from build123d import *

# Parameters (mm, degrees)
EXTRUDE_1_DEPTH          = 7
SKETCH_2_R               = 3.5
CUT_EXTRUDE_2_DEPTH      = 7
FILLET_1_R               = 7
EXTRUDE_2_DEPTH          = 29
SKETCH_4_R               = 7
CUT_EXTRUDE_3_DEPTH      = 30
CUT_EXTRUDE_4_DEPTH      = 6
SKETCH_6_R               = 4
CUT_EXTRUDE_5_DEPTH      = 17
CUT_EXTRUDE_5_DEPTH_BACK = 15
EXTRUDE_3_DEPTH          = 5


with BuildPart() as part:
    # 草图1 → 凸台-拉伸1 (new body)
    with BuildSketch(Plane(origin=(0, 0, 0), x_dir=(1, 0, 0), z_dir=(0, 1, 0))):
        Polygon((0, 0), (27, 0), (27, -37), (-27, -37), (-27, 0), align=None)
    extrude(amount=EXTRUDE_1_DEPTH)

    # 草图2 → 切除-拉伸2 (cut)
    with BuildSketch(Plane(origin=(0, 0, 0), x_dir=(1, 0, 0), z_dir=(0, 1, 0))):
        with Locations((-20, -30)):
            Circle(SKETCH_2_R)
        with Locations((20, -30)):
            Circle(SKETCH_2_R)
    extrude(amount=CUT_EXTRUDE_2_DEPTH, mode=Mode.SUBTRACT)

    # 圆角1
    fillet_1_edges = [part.edges().sort_by_distance(p)[0] for p in [
        (27, 3.5, 37),
        (-27, 3.5, 37),
    ]]
    fillet(fillet_1_edges, radius=FILLET_1_R)

    # 草图3 → 凸台-拉伸2 (add)
    with BuildSketch(Plane(origin=(0, 0, 0), x_dir=(1, 0, 0), z_dir=(0, 1, 0))):
        with BuildLine():
            Line((0, 0), (-12, 0))
            Line((-12, 0), (-12, -14))
            ThreePointArc((-12, -14), (0, -26), (12, -14))
            Line((12, -14), (12, 0))
            Line((12, 0), (0, 0))
        make_face()
    extrude(amount=EXTRUDE_2_DEPTH)

    # 草图4 → 切除-拉伸3 (cut, through all)
    with BuildSketch(Plane(origin=(0, 29, 0), x_dir=(1, 0, 0), z_dir=(0, 1, 0))):
        with Locations((0, -14)):
            Circle(SKETCH_4_R)
    extrude(amount=-CUT_EXTRUDE_3_DEPTH, mode=Mode.SUBTRACT)

    # 草图5 → 切除-拉伸4 (cut)
    with BuildSketch(Plane(origin=(0, 29, 0), x_dir=(1, 0, 0), z_dir=(0, 1, 0))):
        with BuildLine():
            Line((-7, -14), (-12, -14))
            ThreePointArc((-12, -14), (0, -26), (12, -14))
            Line((12, -14), (7, -14))
            ThreePointArc((7, -14), (0, -21), (-7, -14))
        make_face()
    extrude(amount=-CUT_EXTRUDE_4_DEPTH, mode=Mode.SUBTRACT)

    # 草图6 → 切除-拉伸5 (cut, two sides)
    with BuildSketch(Plane.XY.offset(14)) as cut_extrude_5_sk:
        with Locations((0, 23)):
            Circle(SKETCH_6_R)
    extrude(amount=CUT_EXTRUDE_5_DEPTH, mode=Mode.SUBTRACT)
    extrude(cut_extrude_5_sk.sketch, amount=-CUT_EXTRUDE_5_DEPTH_BACK, mode=Mode.SUBTRACT)

    # 草图8 → 凸台-拉伸3 (add)
    with BuildSketch(Plane.XY):
        Polygon((-12, 16), (-18, 7), (-12, 7), align=None)
        Polygon((12, 7), (12, 16), (18, 7), align=None)
    extrude(amount=EXTRUDE_3_DEPTH)


solid = part.part
Could you check a few things on this model? Use its own coordinates, in mm. A direction names the side the tool comes from. Give positions to 0.01 mm unless a question says otherwise; leave off trailing zeros. Order: outer loops, then holes, each group sorted by start corner. A loop starts at its lowest first (then second) coordinate and runs counter-clockwise, first axis right, second up. Notation, with made-up numbers: (-26.75, 18.25) -> (5.25, 18.25) arc R25 cw to (5.25, 47.25) -> close; hole circle Ø8 at (-9, -10). An arc over 180 degrees is marked (long way). Return JSON: item names as keys, results as strings.
1. On a 3-axis mill with a long thin cutter (end or side, diameter ignored), from which of +Z, -Z, +X, -X, +Y, -Y can I reach the whole of each face in a straight line? I mean faces 1 (the cylindrical face through (0, 15, 26)), 2 (the flat face through (-8, 23, 20)), 3 (the flat face through (14, 10, 5)). Say none if no direction works.
Answer list:
{"face 1": "+Z, +Y", "face 2": "+Z, +X, -X, +Y", "face 3": "+Z, +X, +Y"}
2. I need wall thicknesses on line 1 (X direction, y = 2.75, z = 30); line 2 (Z direction, x = -20, y = 3.75); line 3 (Z direction, x = 0, y = 16.5). Which ranges of each line are inside material? Lowest first, please. Write a range as from..to.
Answer list:
{"line 1": "x = -27..-23.5, -16.5..16.5, 23.5..27", "line 2": "z = 0..26.5, 33.5..37", "line 3": "z = 0..7, 21..26"}
3. For pin 1 Ø1.5 at (x, y) = (9, 27) entering from +Z; pin 2 Ø12 at (x, y) = (-21.5, 23.5) entering from +Z; pin 3 Ø3 at (x, y) = (-16.5, 10) entering from +Z; pin 4 Ø6.5 at (x, z) = (-8.5, 22) entering from +Y, each with a flat end and sliding along its axis, tell me the tip position at first contact or that it passes through.
Answer list:
{"pin 1": "stops at z = 14", "pin 2": "passes through", "pin 3": "stops at z = 5", "pin 4": "stops at y = 23"}
4. Imagine slicing it at C-C on z = 18. List the corners of the cut face in (x, y) for me.
Answer list:
{"outline": "(-27, 0) -> (-5.74, 0) -> (-5.74, 23) -> (-11.31, 23) -> (-11.31, 7) -> (-27, 7) -> close; (5.74, 0) -> (27, 0) -> (27, 7) -> (11.31, 7) -> (11.31, 23) -> (5.74, 23) -> close"}
5. Imagine slicing it at A-A on y = 2. List the corners of the cut face in (x, z) for me.
Answer list:
{"outline": "(-27, 0) -> (27, 0) -> (27, 30) arc R7 ccw to (20, 37) -> (-20, 37) arc R7 ccw to (-27, 30) -> close; hole circle Ø7 at (-20, 30); hole circle Ø14 at (0, 14); hole circle Ø7 at (20, 30)"}
6. Thinking about a two-plate mould opening in X: for faces 4 (the flat face through (-9, 26, 14)), 5 (the cylindrical face through (3.815, 24.201, 4.186)), 6 (the cylindrical face through (-20.46, 3.45, 26.53)), 7 (the cylindrical face through (-25, 3.5, 34.9)), which applies, pulls with the +X half, pulls with the -X half, needs draft (parallel to the pull), parting line crosses it, or undercut?
Answer list:
{"face 4": "needs draft", "face 5": "undercut", "face 6": "undercut", "face 7": "pulls with the -X half"}
7. Imagine slicing it at B-B on x = -1.5. List the corners of the cut face in (y, z) for me.
Answer list:
{"outline": "(0, 0) -> (19.29, 0) -> (19.29, 7.16) -> (0, 7.16) -> close; (0, 20.84) -> (19.29, 20.84) -> (19.29, 25.91) -> (7, 25.91) -> (7, 37) -> (0, 37) -> close; (26.71, 0) -> (29, 0) -> (29, 7.16) -> (26.71, 7.16) -> close"}
8. Imagine slicing it at D-D on y = 20. List the corners of the cut face in (x, z) for me.
Answer list:
{"outline": "(-12, 0) -> (-2.65, 0) -> (-2.65, 7.52) arc R7 cw to (-2.65, 20.48) -> (-2.65, 25.7) arc R12 ccw to (-12, 14) -> close; (2.65, 0) -> (12, 0) -> (12, 14) arc R12 ccw to (2.65, 25.7) -> (2.65, 20.48) arc R7 cw to (2.65, 7.52) -> close"}
